Build history of the part. All positions in model axes, mm. Face numbers are marked on the shaded views. A direction names the side the tool comes from. Round coordinates to 2 decimals unless told otherwise and drop trailing zeros. Order: outer loops, then holes, each group sorted by start corner. A loop starts at its lowest first (then second) coordinate and runs counter-clockwise, first axis right, second up. Notation, with made-up numbers: M 64.25,60 L 90.25,60 A18 ccw 90.25,83 Z; hole C -11,26 d5. An arc over 180 degrees is marked long. One line per item, written item: value. Start each with the question number.
Item 1: Band-saw the part on D-D, the plane y = 21.5. Write the cut outline in (x, z).
Item 2: Pin check, flat tips, straight feed: pin 1 (1.2 mm diameter, centred on y = 22.5, z = 55.5, fed in from +X); pin 2 (2 mm diameter, centred on y = 15, z = -41, fed in from +X); pin 3 (3 mm diameter, centred on x = 10, z = 54, fed in from +Y). Stop position of each tip, or through.
Item 3: Band-saw the part on C-C, the plane x = -48. Write the cut outline in (y, z), then the cut area to 3 significant figures.
Item 4: Tool access for the marked faces 1 and 2: list every direction of +Z, -Z, +X, -X, +Y, -Y with a clear straight run to the whole face (end or side of a thin tool).
Item 5: Two-plate mould, pull along Z, no slides. Class the marked faces 3, 4 and 5: +Z half, -Z half, draft (parallel to the pull), parting line (faces both ways), or undercut.
Item 6: Band-saw the part on A-A, the plane y = -2.5. Write the cut outline in (x, z).
Item 7: Probe L1, parallel to Z at x = -12.5, y = 18; L2, parallel to X at y = 7, z = 25; L3, parallel to X at y = 14.5, z = 27. List the from-to ranges inside material, lowest first.
Item 8: Band-saw the part on B-B, the plane z = -27. Write the cut outline in (x, y), then the cut area to 3 significant figures.
```python
from build123d import *

# Parameters (mm, degrees)
SKETCH_1_W           = 75
SKETCH_1_H           = 95
EXTRUDE_1_DEPTH      = 25
SHELL_1_T            = -2
SKETCH_2_W           = 75
SKETCH_2_H           = 25
EXTRUDE_2_DEPTH      = 4
SKETCH_3_W           = 75
SKETCH_3_H           = 25
EXTRUDE_3_DEPTH      = 4
CUT_EXTRUDE_2_DEPTH  = 4
CUT_EXTRUDE_START    = -4
CUT_EXTRUDE_3_DEPTH  = 4
SKETCH_6_R           = 1.6
CUT_EXTRUDE_4_DEPTH  = 150
SKETCH_7_W           = 95
SKETCH_7_H           = 12.742640687
CUT_EXTRUDE_5_DEPTH  = 2
CUT_EXTRUDE_6_DEPTH  = 4
CUT_EXTRUDE_7_DEPTH  = 4
CUT_EXTRUDE_9_DEPTH  = 150
SKETCH_11_W          = 75
SKETCH_11_H          = 103
EXTRUDE_4_DEPTH      = 6
SKETCH_12_W          = 71
SKETCH_12_H          = 91
CUT_EXTRUDE_10_DEPTH = 6


with BuildPart() as part:
    # 草图1 → 凸台-拉伸1 (new body)
    with BuildSketch(Plane(origin=(0, 0, 0), x_dir=(1, 0, 0), z_dir=(0, 1, 0))):
        with Locations((-21.666666667, -5.700239808)):
            Rectangle(SKETCH_1_W, SKETCH_1_H)
    extrude(amount=EXTRUDE_1_DEPTH)

    # 抽壳1
    shell_1_openings = [part.faces().sort_by_distance(p)[0] for p in [
        (-21.666666667, 25, 5.700239808),
    ]]
    offset(amount=SHELL_1_T, openings=shell_1_openings, kind=Kind.INTERSECTION)

    # 草图2 → 凸台-拉伸2 (add)
    with BuildSketch(Plane.XY.offset(53.200239808)):
        with Locations((-21.666666667, 12.5)):
            Rectangle(SKETCH_2_W, SKETCH_2_H)
    extrude(amount=EXTRUDE_2_DEPTH)

    # 草图3 → 凸台-拉伸3 (add)
    with BuildSketch(Plane(origin=(0, 0, -41.799760192), x_dir=(-1, 0, 0), z_dir=(0, 0, -1))):
        with Locations((21.666666667, 12.5)):
            Rectangle(SKETCH_3_W, SKETCH_3_H)
    extrude(amount=EXTRUDE_3_DEPTH)

    # 草图4 → 切除-拉伸2 (cut)
    with BuildSketch(Plane(origin=(0, 0, -45.799760192), x_dir=(-1, 0, 0), z_dir=(0, 0, -1))):
        with BuildLine():
            Line((-16.833333333, 26), (-16.833333333, 16.5))
            ThreePointArc((-16.833333333, 16.5), (-7.333333333, 7), (2.166666667, 16.5))
            Line((2.166666667, 16.5), (2.166666667, 26))
            Line((2.166666667, 26), (-16.833333333, 26))
        make_face()
    extrude(amount=-CUT_EXTRUDE_2_DEPTH, mode=Mode.SUBTRACT)

    # 草图5 → 切除-拉伸3 (cut)
    with BuildSketch(Plane.XY.offset(57.200239808).offset(CUT_EXTRUDE_START)):
        with BuildLine():
            Line((-2.166666667, 26), (-2.166666667, 16.5))
            ThreePointArc((-2.166666667, 16.5), (7.333333333, 7), (16.833333333, 16.5))
            Line((16.833333333, 16.5), (16.833333333, 26))
            Line((16.833333333, 26), (-2.166666667, 26))
        make_face()
    extrude(amount=CUT_EXTRUDE_3_DEPTH, mode=Mode.SUBTRACT)

    # 草图6 → 切除-拉伸4 (cut)
    with BuildSketch(Plane.XY.offset(53.200239808)):
        with Locations((6.833333333, 16.5)):
            Circle(SKETCH_6_R)
    extrude(amount=-CUT_EXTRUDE_4_DEPTH, mode=Mode.SUBTRACT)

    # 草图7 → 切除-拉伸5 (cut)
    with BuildSketch(Plane(origin=(15.833333333, 0, 0), x_dir=(0, 0, -1), z_dir=(1, 0, 0))):
        with Locations((-5.700239808, 18.628679657)):
            Rectangle(SKETCH_7_W, SKETCH_7_H)
    extrude(amount=-CUT_EXTRUDE_5_DEPTH, mode=Mode.SUBTRACT)

    # 草图8 → 切除-拉伸6 (cut)
    with BuildSketch(Plane(origin=(0, 0, -45.799760192), x_dir=(-1, 0, 0), z_dir=(0, 0, -1))):
        Polygon((-7.333333333, 7), (-15.833333333, 7), (-15.833333333, 12.257359313), align=None)
    extrude(amount=-CUT_EXTRUDE_6_DEPTH, mode=Mode.SUBTRACT)

    # 草图9 → 切除-拉伸7 (cut)
    with BuildSketch(Plane.XY.offset(57.200239808)):
        Polygon((7.333333333, 7), (15.833333333, 7), (15.833333333, 12.257359313), align=None)
    extrude(amount=-CUT_EXTRUDE_7_DEPTH, mode=Mode.SUBTRACT)

    # 草图10 → 切除-拉伸9 (cut)
    with BuildSketch(Plane(origin=(0, 0, -41.799760192), x_dir=(-1, 0, 0), z_dir=(0, 0, -1))):
        with BuildLine():
            ThreePointArc((-13.833333333, 19), (-12.07597402, 23.242640687), (-7.833333333, 25))
            Line((-7.833333333, 25), (-13.833333333, 25))
            Line((-13.833333333, 25), (-13.833333333, 19))
        make_face()
    extrude(amount=-CUT_EXTRUDE_9_DEPTH, mode=Mode.SUBTRACT)

    # 草图11 → 凸台-拉伸4 (add)
    with BuildSketch(Plane.XZ):
        with Locations((-21.666666667, 5.700239808)):
            Rectangle(SKETCH_11_W, SKETCH_11_H)
    extrude(amount=EXTRUDE_4_DEPTH)

    # 草图12 → 切除-拉伸10 (cut)
    with BuildSketch(Plane(origin=(0, 2, 0), x_dir=(1, 0, 0), z_dir=(0, 1, 0))):
        with Locations((-21.666666667, -5.700239808)):
            Rectangle(SKETCH_12_W, SKETCH_12_H)
    extrude(amount=-CUT_EXTRUDE_10_DEPTH, mode=Mode.SUBTRACT)


solid = part.part
```
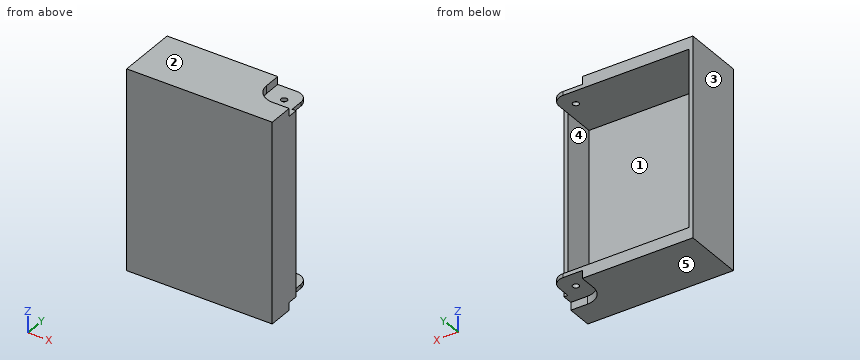
Output:
1. outline: M -59.17,-45.8 L -2.17,-45.8 L -2.17,-41.8 L 13.29,-41.8 L 13.29,-39.8 L -57.17,-39.8 L -57.17,51.2 L 13.29,51.2 L 13.29,53.2 L -2.17,53.2 L -2.17,57.2 L -59.17,57.2 Z
2. pin 1: stops at x = -2.17
2. pin 2: stops at x = 13.83
2. pin 3: stops at y = 24.93
3. outline: M -6,-45.8 L 25,-45.8 L 25,-39.8 L -4,-39.8 L -4,51.2 L 25,51.2 L 25,57.2 L -6,57.2 Z
3. area: 554 mm²
4. face 1: +Y
4. face 2: +Z, +X, -X, +Y, -Y
5. face 3: draft
5. face 4: undercut
5. face 5: -Z half
6. outline: M -59.17,-45.8 L 15.83,-45.8 L 15.83,57.2 L -59.17,57.2 Z; hole M -57.17,-39.8 L 13.83,-39.8 L 13.83,51.2 L -57.17,51.2 Z
7. L1: z = -45.8 to -39.8, 51.2 to 57.2
7. L2: x = -59.17 to -57.17, 13.83 to 15.83
7. L3: x = -59.17 to -57.17
8. outline: M -59.17,-6 L 15.83,-6 L 15.83,12.26 L 13.83,12.26 L 13.83,-4 L -57.17,-4 L -57.17,25 L -59.17,25 Z
8. area: 241 mm²
